Can you work these out from the model? Positions are in its coordinate system, mm. Face numbers are marked on the shaded views. A direction names the side the tool comes from. Coordinates: 2 decimals unless noted, no trailing zeros. Write each loop counter-clockwise with the first axis right and the second up, starting at its lowest first coordinate (ties: lowest second). Pieces come first, ordered by that corner, then holes. Notation, with made-up numbers: (-8.75, 3) - (26.25, 3) arc R21 ccw to (26.25, 10) - close; hole circle Ø11 at (80.25, -12.5). An arc over 180 degrees is marked (long way). Use one line per item in the form item = value. Start each with the question number.
(1) If we section it at D-D on z = 1.5: Please give me the cut outline in (x, y), then the cut area to 3 significant figures.
(2) If we section it at C-C on y = 0: Please give me the cut outline in (x, z).
(3) On a 3-axis mill with a long thin cutter (end or side, diameter ignored), from which of +Z, -Z, +X, -X, +Y, -Y can I reach the whole of each face in a straight line? I mean the marked faces 4, 5 and 6. Say none if no direction works.
(4) If I drill on probe 1 along Y at (x, z) = (0, 2.2); probe 2 along Z at (x, y) = (-2.5, 1.75); probe 3 along X at (y, z) = (2.5, 8.75), over which ranges is the centre line in solid material (lowest first)? Write a range as from..to.
(5) If we section it at B-B on z = 8.5: Please give me the cut outline in (x, y), then the cut area to 3 significant figures.
(6) Thinking about a two-plate mould opening in X: for the marked faces 1, 2 and 3, which applies, pulls with the +X half, pulls with the -X half, needs draft (parallel to the pull), parting line crosses it, or undercut?
(7) If we section it at A-A on x = 0: Please give me the cut outline in (y, z).
```python
from build123d import *

# Parameters (mm, degrees)
SKETCH_W     = 14
SKETCH_H     = 8
SKETCH_R     = 2.3
PAD_DEPTH    = 3
SKETCH001_W  = 2
SKETCH001_H  = 8
PAD001_DEPTH = 10
SKETCH003_W  = 8
SKETCH003_H  = 2
PAD003_DEPTH = 3.5
SKETCH004_W  = 8
SKETCH004_H  = 2
PAD004_DEPTH = 3.5


with BuildPart() as pad001:
    # Sketch → Pad (new body)
    with BuildSketch(Plane.XY):
        Rectangle(SKETCH_W, SKETCH_H)
        Circle(SKETCH_R, mode=Mode.SUBTRACT)
    extrude(amount=PAD_DEPTH)

    # Sketch001 → Pad001 (new body)
    with BuildSketch(Plane.XY.offset(3)):
        with Locations((-6, 0)):
            Rectangle(SKETCH001_W, SKETCH001_H)
        with Locations((6, 0)):
            Rectangle(SKETCH001_W, SKETCH001_H)
    extrude(amount=PAD001_DEPTH)


with BuildPart() as pad003:
    # Pad003 base: copy of Pad001
    add(pad001.part)

    # Sketch003 → Pad003 (new body)
    with BuildSketch(Plane(origin=(5, 0, 0), x_dir=(0, -1, 0), z_dir=(-1, 0, 0))):
        with Locations((0, 12)):
            Rectangle(SKETCH003_W, SKETCH003_H)
    extrude(amount=PAD003_DEPTH)


with BuildPart() as fusion:
    # Pad004 base: copy of Pad001
    add(pad001.part)

    # Sketch004 → Pad004 (new body)
    with BuildSketch(Plane.YZ.offset(-5)):
        with Locations((0, 12)):
            Rectangle(SKETCH004_W, SKETCH004_H)
    extrude(amount=PAD004_DEPTH)

    # Fusion: union Pad003
    add(pad003.part)


solid = fusion.part
```
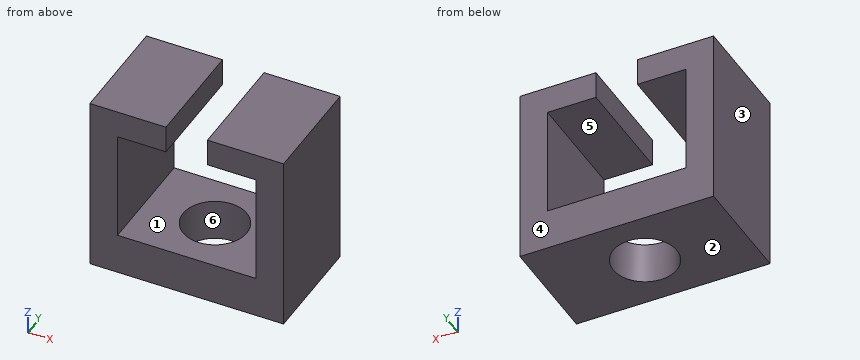
Reported:
q1.outline = (-7, -4) - (7, -4) - (7, 4) - (-7, 4) - close; hole circle Ø4.6 at (0, 0)
q1.area = 95.4 mm2
q2.outline = (-7, 0) - (-2.3, 0) - (-2.3, 3) - (-5, 3) - (-5, 11) - (-1.5, 11) - (-1.5, 13) - (-7, 13) - close; (1.5, 11) - (5, 11) - (5, 3) - (2.3, 3) - (2.3, 0) - (7, 0) - (7, 13) - (1.5, 13) - close
q3.face_4 = +Z, -Z, +X, -X, +Y
q3.face_5 = +Y, -Y
q3.face_6 = -Z
q4.probe_1 = -4..-2.3, 2.3..4
q4.probe_2 = 0..3, 11..13
q4.probe_3 = -7..-5, 5..7
q5.outline = (-7, -4) - (-5, -4) - (-5, 4) - (-7, 4) - close; (5, -4) - (7, -4) - (7, 4) - (5, 4) - close
q5.area = 32.0 mm2
q6.face_1 = undercut
q6.face_2 = needs draft
q6.face_3 = pulls with the -X half
q7.outline = (-4, 0) - (-2.3, 0) - (-2.3, 3) - (-4, 3) - close; (2.3, 0) - (4, 0) - (4, 3) - (2.3, 3) - close
